Geometry: final body of the model. Coordinates: model frame, mm. A direction names the side the tool comes from. Give positions to 0.01 mm unless a question says otherwise; leave off trailing zeros. One line per item, written item: value. Start each with the question number.
```python
from build123d import *

# Parameters (mm, degrees)
F1_DEPTH = 10.16
F2_R     = 5.08
F3_R     = 5.07999


# Not quite as in the source:
# - a fillet or chamfer is up to 0.001 mm smaller than in the source, because OpenCascade refuses the exact size


with BuildPart() as f1:
    # F0 (on Top) → F1 (new body)
    with BuildSketch(Plane.XY):
        Polygon((19.1086118392, 0.1538227311), (-9.6875203124, 16.4716319182), (-9.4210915267, -16.6254546493), align=None)
    extrude(amount=F1_DEPTH)

    # F2
    f2_edges = [f1.edges().sort_by_distance(p)[0] for p in [
        (-9.421092, -16.625455, 5.08),
        (19.108612, 0.153823, 5.08),
        (-9.68752, 16.471632, 5.08),
    ]]
    fillet(f2_edges, radius=F2_R)

    # F3 (radius 5.08 in the source; OpenCascade refuses exactly that, so slightly less here)
    f3_edges = [f1.edges().sort_by_distance(p)[0] for p in [
        (4.84376, -8.235816, 0),
        (-6.916588, -12.205742, 0),
        (14.028776, 0.11293, 0),
        (-9.554306, -0.076911, 0),
        (4.710546, 8.312727, 0),
        (-7.112189, 12.092812, 0),
        (4.84376, -8.235816, 10.16),
        (-6.916588, -12.205742, 10.16),
        (14.028776, 0.11293, 10.16),
        (-9.554306, -0.076911, 10.16),
        (4.710546, 8.312727, 10.16),
        (-7.112189, 12.092812, 10.16),
    ]]
    fillet(f3_edges, radius=F3_R)


solid = f1.part
```
1. Pin query (flat end, axial travel): P1, Ø4, axis at x = 9, y = -10, coming from the -Z side; P2, Ø8, axis at x = 11, y = 6.5, coming from the -Z side; P3, Ø4, axis at x = -3, y = -10.5, coming from the +Z side; P4, Ø5, axis at x = -3, z = 4, coming from the +Y side. Return the tip coordinate at first contact, or that it passes through.
2. Access query for faces 1 (the cylindrical face through (-8.03, -0.17, 1.45)), 2 (the flat face through (1, 0, 10.16)), 3 (the cylindrical face through (-8.03, -0.17, 8.71)). Directions: +Z, -Z, +X, -X, +Y, -Y. A direction counts if a zero-diameter tool reaches every point of the face in a straight line with its end or side. Return the directions, or none.
3. Material intervals for L1, parallel to Z at x = -8.5, y = 5.75; L2, parallel to Y at x = 10.75, z = 4.5, sorted ascending. Write a range as [from, to].
Answers follow:
1. P1: passes through
1. P2: stops at z = 0.72
1. P3: stops at z = 10.05
1. P4: stops at y = 12.79
2. face 1: -Z, -X, -Y
2. face 2: +Z, +X, -X, +Y, -Y
2. face 3: +Z, -X, -Y
3. L1: z = [1.92, 8.24]
3. L2: y = [-4.72, 4.85]
